The listing builds one solid part. Answer for the finished solid, in the listing's coordinates (mm). A direction names the side the tool comes from. Round coordinates to 2 decimals unless told otherwise and drop trailing zeros. Write each loop counter-clockwise with the first axis right and the second up, starting at its lowest first coordinate (ties: lowest second). Pieces come first, ordered by that corner, then holes.
from build123d import *

# Parameters (mm, degrees)
SKETCH1_W           = 195
SKETCH1_H           = 67
BOSS_EXTRUDE1_DEPTH = 20
CUT_EXTRUDE1_DEPTH  = 20
CUT_EXTRUDE2_DEPTH  = 120.980206701
CUT_EXTRUDE3_START  = -13
SKETCH4_W           = 3.612655346
SKETCH4_H           = 3
CUT_EXTRUDE3_DEPTH  = 13
SKETCH6_R           = 2.5
CUT_EXTRUDE4_DEPTH  = 106.016665344
SKETCH7_W           = 37
SKETCH7_H           = 35
CUT_EXTRUDE5_DEPTH  = 1.5
CUT_EXTRUDE6_DEPTH  = 18.5


with BuildPart() as part:
    # Sketch1 → Boss-Extrude1 (new body)
    with BuildSketch(Plane(origin=(0, 0, 0), x_dir=(1, 0, 0), z_dir=(0, 1, 0))):
        Rectangle(SKETCH1_W, SKETCH1_H)
    extrude(amount=BOSS_EXTRUDE1_DEPTH)

    # Sketch2 → Cut-Extrude1 (cut)
    with BuildSketch(Plane.XZ):
        with BuildLine():
            Line((97.5, -3.219751644), (97.5, 33.5))
            Line((97.5, 33.5), (88.5, 33.5))
            ThreePointArc((88.5, 33.5), (95.217186872, 15.683556008), (97.5, -3.219751644))
        make_face()
        with BuildLine():
            Line((97.5, -33.5), (97.5, -3.219751644))
            ThreePointArc((97.5, -3.219751644), (95.985558513, -18.65423771), (91.5, -33.5))
            Line((91.5, -33.5), (97.5, -33.5))
        make_face()
        with BuildLine():
            ThreePointArc((-88, -33.5), (-95.08607052, -15.861694529), (-97.5, 2.992884749))
            Line((-97.5, 2.992884749), (-97.5, -33.5))
            Line((-97.5, -33.5), (-88, -33.5))
        make_face()
        with BuildLine():
            ThreePointArc((-97.5, 2.992884749), (-95.856964648, 18.588830376), (-91, 33.5))
            Line((-91, 33.5), (-97.5, 33.5))
            Line((-97.5, 33.5), (-97.5, 2.992884749))
        make_face()
    extrude(amount=-CUT_EXTRUDE1_DEPTH, mode=Mode.SUBTRACT)

    # Sketch3 → Cut-Extrude2 (cut, through all)
    with BuildSketch(Plane(origin=(0, 0, 33.5), x_dir=(-1, 0, 0), z_dir=(0, 0, -1))):
        Polygon((63.2, 20), (63.2, 9.6), (40.2, 9.6), (40.2, 5.6), (-61.8, 5.6), (-61.8, 9.6), (-97.5, 9.6), (-97.5, 20), align=None)
    extrude(amount=CUT_EXTRUDE2_DEPTH, mode=Mode.SUBTRACT)

    # Sketch4 → Cut-Extrude3 (cut)
    with BuildSketch(Plane(origin=(0, 20, 0), x_dir=(1, 0, 0), z_dir=(0, 1, 0)).offset(CUT_EXTRUDE3_START)):
        with BuildLine():
            Line((-63.2, 30.5), (-63.2, 33.5))
            Line((-63.2, 33.5), (-88, 33.5))
            ThreePointArc((-88, 33.5), (-88.810680862, 32.008999469), (-89.587344654, 30.5))
            Line((-89.587344654, 30.5), (-63.2, 30.5))
        make_face()
        with Locations((-61.393672327, 32)):
            Rectangle(SKETCH4_W, SKETCH4_H)
        with BuildLine():
            Line((-63.2, -33.5), (-63.2, -30.5))
            Line((-63.2, -30.5), (-92.261692194, -30.5))
            ThreePointArc((-92.261692194, -30.5), (-91.647155152, -32.006859002), (-91, -33.5))
            Line((-91, -33.5), (-63.2, -33.5))
        make_face()
        with Locations((-61.393672327, -32)):
            Rectangle(SKETCH4_W, SKETCH4_H)
    extrude(amount=CUT_EXTRUDE3_DEPTH, mode=Mode.SUBTRACT)

    # Sketch6 → Cut-Extrude4 (cut, through all)
    with BuildSketch(Plane.XZ):
        with Locations(Location((-28.1, -9, 0), (0, 0, 270))):
            Circle(SKETCH6_R)
        with Locations(Location((-8.2, -8.3, 0), (0, 0, 270))):
            Circle(SKETCH6_R)
        with Locations(Location((-18.7, 8.7, 0), (0, 0, 270))):
            Circle(SKETCH6_R)
        with Locations(Location((-76.2, 22, 0), (0, 0, 270))):
            Circle(SKETCH6_R)
        with Locations(Location((-78.2, 0.1, 0), (0, 0, 270))):
            Circle(SKETCH6_R)
        with Locations(Location((-73.2, -22.3, 0), (0, 0, 270))):
            Circle(SKETCH6_R)
        with Locations(Location((65.3, -20, 0), (0, 0, 270))):
            Circle(SKETCH6_R)
        with Locations(Location((74.1, -1.7, 0), (0, 0, 270))):
            Circle(SKETCH6_R)
        with Locations(Location((68.3, 21.5, 0), (0, 0, 270))):
            Circle(SKETCH6_R)
    extrude(amount=-CUT_EXTRUDE4_DEPTH, mode=Mode.SUBTRACT)

    # Sketch7 → Cut-Extrude5 (cut)
    with BuildSketch(Plane(origin=(0, 5.6, 0), x_dir=(1, 0, 0), z_dir=(0, 1, 0))):
        with Locations((5.3, -16)):
            Rectangle(SKETCH7_W, SKETCH7_H)
    extrude(amount=-CUT_EXTRUDE5_DEPTH, mode=Mode.SUBTRACT)

    # Sketch8 → Cut-Extrude6 (cut)
    with BuildSketch(Plane(origin=(0, 20, 0), x_dir=(1, 0, 0), z_dir=(0, 1, 0))):
        with BuildLine():
            Line((37.096152423, 33.5), (31.9, 33.5))
            Line((31.9, 33.5), (31.9, 30.5))
            ThreePointArc((31.9, 30.5), (34.9, 31.303847577), (37.096152423, 33.5))
        make_face()
        with BuildLine():
            Line((31.9, 33.5), (26.703847577, 33.5))
            ThreePointArc((26.703847577, 33.5), (28.9, 31.303847577), (31.9, 30.5))
            Line((31.9, 30.5), (31.9, 33.5))
        make_face()
    extrude(amount=-CUT_EXTRUDE6_DEPTH, mode=Mode.SUBTRACT)


solid = part.part
1. Straight lines are drawn through the part: line 1 along X through (y, z) = (7.25, 21.5); line 2 along Y through (x, z) = (30.5, -24); line 3 along X through (y, z) = (4, -8.3). For each, find the intervals that lie inside material, in ascending order.
Geometry says:
line 1: x = -95.18 to -78.65, -73.75 to -40.2, 61.8 to 65.8, 70.8 to 93.55
line 2: y = 0 to 5.6
line 3: x = -96.64 to -30.5, -25.7 to -10.7, -5.7 to 97.34
2. Section A-A on y = 15.75 is taken. Determine the outline of the cut face in (x, z), plus the area to 3 significant figures.
Geometry says:
outline: (-92.26, 30.5) arc R74.84 ccw to (-89.59, -30.5) - (-63.2, -30.5) - (-63.2, 30.5) - close; hole circle Ø5 at (-78.2, 0.1); hole circle Ø5 at (-76.2, 22); hole circle Ø5 at (-73.2, -22.3)
area: 1,900 mm2
3. Section D-D on z = 8.7 is taken. Determine the outline of the cut face in (x, y).
Geometry says:
outline: (-97.28, 0) - (-21.2, 0) - (-21.2, 5.6) - (-40.2, 5.6) - (-40.2, 9.6) - (-63.2, 9.6) - (-63.2, 20) - (-97.28, 20) - close; (-16.2, 0) - (96.6, 0) - (96.6, 9.6) - (61.8, 9.6) - (61.8, 5.6) - (23.8, 5.6) - (23.8, 4.1) - (-13.2, 4.1) - (-13.2, 5.6) - (-16.2, 5.6) - close
4. Section C-C on z = -9 is taken. Determine the outline of the cut face in (x, y), plus the area to 3 significant figures.
Geometry says:
outline: (-96.53, 0) - (-30.6, 0) - (-30.6, 5.6) - (-40.2, 5.6) - (-40.2, 9.6) - (-63.2, 9.6) - (-63.2, 20) - (-96.53, 20) - close; (-25.6, 0) - (-10.6, 0) - (-10.6, 5.6) - (-25.6, 5.6) - close; (-5.8, 0) - (97.29, 0) - (97.29, 9.6) - (61.8, 9.6) - (61.8, 5.6) - (-5.8, 5.6) - close
area: 1,740 mm2
5. Section B-B on x = -8.2 is taken. Determine the outline of the cut face in (y, z).
Geometry says:
outline: (0, -33.5) - (5.6, -33.5) - (5.6, -10.8) - (0, -10.8) - close; (0, -5.8) - (5.6, -5.8) - (5.6, -1.5) - (4.1, -1.5) - (4.1, 33.5) - (0, 33.5) - close
6. Given pin 1 (6 mm diameter, centred on x = -19, z = -15.5, fed in from +Y); pin 2 (8 mm diameter, centred on x = 3, z = 19, fed in from +Y); pin 3 (1.2 mm diameter, centred on y = 5, z = 16, fed in from -X), each flat-ended and moving along its own axis, determine where each tip first touches the part or whether it passes through.
Geometry says:
pin 1: stops at y = 5.6
pin 2: stops at y = 4.1
pin 3: stops at x = -96.46
7. A tool of negligible diameter and unlimited length cuts with its end or side. For faces 4 (the face through (-52, 9.6, 0)), 5 (the face through (-76, 13, 30.5)), 6 (the face through (5, 4.1, 16)), 7 (the face through (10, 5.6, -7)), from which of +Z, -Z, +X, -X, +Y, -Y can it reach the whole face along a straight path? Write none if from no direction.
Geometry says:
face 4: +Z, -Z, +X, +Y
face 5: +Z, -X, +Y
face 6: +Z, +Y
face 7: +Z, -Z, +Y
8. For a pull along Z with two mould halves and no side action, classify faces 1 (the face through (-6.09, 2.76, -9.64)), 2 (the face through (0, 4, -33.5)), 3 (the face through (79, 9.6, 0)) as released by +Z, released by -Z, zero draft, split by the parting line, or undercut.
Geometry says:
face 1: undercut
face 2: released by -Z
face 3: zero draft
